Input: part model. Units: mm. Frame: model coordinates. A direction names the side the tool comes from. Coordinates: 2 decimals unless noted, no trailing zeros. Write each loop counter-clockwise with the first axis right and the second up, starting at its lowest first coordinate (ties: lowest second). Pieces come first, ordered by that corner, then holes. Notation, with made-up numbers: M -1.5,-2 L 33.5,-2 A34 ccw 33.5,30 Z; hole C 71,65 d1. An arc over 180 degrees is marked long. Use one line per item in the form item = value.
from build123d import *

# Parameters (mm, degrees)
AUFSATZ_LINEAR_AUSTRAGEN1_DEPTH = 2.5
AUFSATZ_LINEAR_AUSTRAGEN2_DEPTH = 3.5
SKIZZE3_R                       = 1.5
SCHNITT_LINEAR_AUSTRAGEN1_DEPTH = 7


with BuildPart() as part:
    # Skizze1 → Aufsatz-Linear austragen1 (new body)
    with BuildSketch(Plane(origin=(0, 0, 0), x_dir=(1, 0, 0), z_dir=(0, 1, 0))):
        with BuildLine():
            Line((0, 0), (0, 20))
            ThreePointArc((0, 20), (5, 25), (10, 20))
            Line((10, 20), (10, 0))
            Line((10, 0), (0, 0))
        make_face()
    extrude(amount=AUFSATZ_LINEAR_AUSTRAGEN1_DEPTH)

    # Skizze2 → Aufsatz-Linear austragen2 (add)
    with BuildSketch(Plane(origin=(0, 2.5, 0), x_dir=(1, 0, 0), z_dir=(0, 1, 0))):
        with BuildLine():
            Line((0, 20), (0, 15.3))
            Line((0, 15.3), (10, 15.3))
            Line((10, 15.3), (10, 20))
            ThreePointArc((10, 20), (5, 25), (0, 20))
        make_face()
    extrude(amount=AUFSATZ_LINEAR_AUSTRAGEN2_DEPTH)

    # Skizze3 → Schnitt-Linear austragen1 (cut, through all)
    with BuildSketch(Plane(origin=(0, 6, 0), x_dir=(1, 0, 0), z_dir=(0, 1, 0))):
        with Locations((5, 20)):
            Circle(SKIZZE3_R)
    extrude(amount=-SCHNITT_LINEAR_AUSTRAGEN1_DEPTH, mode=Mode.SUBTRACT)


solid = part.part
(1) Section query B-B on y = 4.75. Return the cut outline in (x, z).
Computed:
outline = M 0,-20 A5 ccw 10,-20 L 10,-15.3 L 0,-15.3 Z; hole C 5,-20 d3
(2) Set-up query: faces 1 (the flat face through (5, 2.5, -8)), 2 (the cylindrical face through (5, 3, -25)). Return all of +Z, -Z, +X, -X, +Y, -Y with unobstructed straight access to the full face (end or side cutting, diameter ignored); none if empty.
Computed:
face_1 = +Z, +X, -X, +Y
face_2 = -Z, +Y, -Y
(3) Line query: probe 1 along X at (y, z) = (2.05, -20); probe 2 along Z at (x, y) = (5, 2); probe 3 along Z at (x, y) = (5, 4.65). Output: solid intervals per line, ascending.
Computed:
probe_1 = 0 to 3.5, 6.5 to 10
probe_2 = -25 to -21.5, -18.5 to 0
probe_3 = -25 to -21.5, -18.5 to -15.3
(4) First-contact query: pin 1 Ø3 at (x, z) = (5.5, -10) entering from +Y; pin 2 Ø1 at (x, y) = (5.5, 4.5) entering from +Z. Flat tips, straight axial feed; report the tip coordinate or a pass-through.
Computed:
pin_1 = 2.5
pin_2 = -15.3
(5) Section query D-D on z = -9.25. Return the cut outline in (x, y), plus the area to 3 significant figures.
Computed:
outline = M 0,0 L 10,0 L 10,2.5 L 0,2.5 Z
area = 25.0 mm^2
(6) Section query A-A on x = 5. Return the cut outline in (y, z), plus the area to 4 significant figures.
Computed:
outline = M 0,-25 L 6,-25 L 6,-21.5 L 0,-21.5 Z; M 0,-18.5 L 6,-18.5 L 6,-15.3 L 2.5,-15.3 L 2.5,0 L 0,0 Z
area = 78.45 mm^2
(7) Pull-direction query (Z, two-part tool) for faces 3 (the flat face through (10, 2, -12)), 4 (the cylindrical face through (4.805, 3.042, -21.487)), 5 (the flat face through (5, 4, -15.3)); classes: pulls with the +Z half, pulls with the -Z half, needs draft (parallel to the pull), parting line crosses it, or undercut.
Computed:
face_3 = needs draft
face_4 = undercut
face_5 = pulls with the +Z half
(8) Section query C-C on z = -21.25. Return the cut outline in (x, y).
Computed:
outline = M 0.16,0 L 4.17,0 L 4.17,6 L 0.16,6 Z; M 5.83,0 L 9.84,0 L 9.84,6 L 5.83,6 Z
